Input: part model. Units: mm. Frame: model coordinates. A direction names the side the tool comes from. Coordinates: 2 decimals unless noted, no trailing zeros. Order: outer loops, then holes, each group sorted by start corner. A loop starts at its lowest first (then second) coordinate and runs counter-clockwise, first axis right, second up. Notation, with made-up numbers: (46, -37.75) -> (103, -37.75) arc R28 cw to (103, -18.75) -> close; hole circle Ø5 at (29, -31.75). An arc over 180 degrees is marked (long way). Write each question's results on one line, items separated by ' | '.
```python
from build123d import *

# Parameters (mm, degrees)
F0_R     = 3
F0_R_2   = 1.25
F1_DEPTH = 30
F2_DEPTH = 9
F3_R     = 1.25
F4_DEPTH = 9


with BuildPart() as f1:
    # F0 (on Top) → F1 (new body)
    with BuildSketch(Plane.XY):
        Circle(F0_R)
        Circle(F0_R_2, mode=Mode.SUBTRACT)
        Circle(F0_R_2)
    extrude(amount=F1_DEPTH)

    # F0 (on Top) → F2 (cut)
    with BuildSketch(Plane.XY):
        Circle(F0_R_2)
    extrude(amount=F2_DEPTH, mode=Mode.SUBTRACT)

    # F3 (on face) → F4 (cut)
    with BuildSketch(Plane.XY.offset(30)):
        Circle(F3_R)
    extrude(amount=-F4_DEPTH, mode=Mode.SUBTRACT)


solid = f1.part
```
(1) Pin query (flat end, axial travel): P1, Ø2, axis at x = 0, y = 1, coming from the -Z side; P2, Ø2, axis at x = 0, y = 0, coming from the -Z side; P3, Ø2, axis at y = -1.5, z = 5.5, coming from the +X side; P4, Ø2, axis at x = 0, y = 0, coming from the +Z side. Return the tip coordinate at first contact, or that it passes through.
Return value:
P1: z = 0 | P2: z = 9 | P3: x = 2.96 | P4: z = 21
(2) Mould query, pull axis Y, two halves, no side actions, for faces 4 (the face through (0, 0, 9)), 5 (the face through (1, -1, 0)), 6 (the face through (-3, 0, 15)). Classes: +Y half, -Y half, draft (parallel to the pull), parting line (faces both ways), or undercut.
Return value:
face 4: undercut | face 5: draft | face 6: parting line
(3) Cut plane D-D, the plane z = 15.75. Return loops of the section in (x, y), plus the area to 3 significant figures.
Return value:
outline: circle Ø6 at (0, 0) | area: 28.3 mm2
(4) Reachability of faces 1 (the face through (1, -1, 30)), 2 (the face through (-0.27, -1.22, 4.44)), 3 (the face through (0, 0, 21)) from +Z, -Z, +X, -X, +Y, -Y: full face, straight path, thin tool, end or side. Return the list, or none.
Return value:
face 1: +Z, +X, -X, +Y, -Y | face 2: -Z | face 3: +Z
(5) Cut plane C-C, the plane z = 5. Return loops of the section in (x, y).
Return value:
outline: circle Ø6 at (0, 0); hole circle Ø2.5 at (0, 0)
(6) Line query: line 1 along Y through (x, z) = (0, 26.75); line 2 along Z through (x, y) = (0.5, 0.3); line 3 along Y through (x, z) = (1.1, 8.75). Output: solid intervals per line, ascending. Write a range as from..to.
Return value:
line 1: -3..-1.25, 1.25..3 | line 2: 9..21 | line 3: -2.79..-0.59, 0.59..2.79
(7) Cut plane A-A, the plane y = 0. Return loops of the section in (x, z), plus the area to 3 significant figures.
Return value:
outline: (-3, 0) -> (-1.25, 0) -> (-1.25, 9) -> (1.25, 9) -> (1.25, 0) -> (3, 0) -> (3, 30) -> (1.25, 30) -> (1.25, 21) -> (-1.25, 21) -> (-1.25, 30) -> (-3, 30) -> close | area: 135 mm2
